from build123d import *

# Parameters (mm, degrees)
F1_DEPTH = 15
F2_R     = 3
F3_R     = 3
F4_R     = 3


with BuildPart() as f1:
    # F0 (on Front) → F1 (new body)
    with BuildSketch(Plane.XZ):
        with BuildLine():
            Line((-16, 27.1340573728), (-16, -16.8659426272))
            Line((-16, -16.8659426272), (-16, -22.8659426272))
            Line((-16, -22.8659426272), (6, -22.8659426272))
            Line((6, -22.8659426272), (6, 27.1340573728))
            Line((6, 27.1340573728), (15, 27.1340573728))
            Line((15, 27.1340573728), (21, 27.1340573728))
            Line((21, 27.1340573728), (21, 49.1340573728))
            Line((21, 49.1340573728), (6, 49.1340573728))
            Line((6, 49.1340573728), (6, 64.1340573728))
            Line((6, 64.1340573728), (0.3713240896, 64.1340573728))
            ThreePointArc((0.3713240896, 64.1340573728), (-5, 58.7627332832), (-10.3713240896, 64.1340573728))
            Line((-10.3713240896, 64.1340573728), (-16, 64.1340573728))
            Line((-16, 64.1340573728), (-16, 49.1340573728))
            Line((-16, 49.1340573728), (-31, 49.1340573728))
            Line((-31, 49.1340573728), (-31, 27.1340573728))
            Line((-31, 27.1340573728), (-25, 27.1340573728))
            Line((-25, 27.1340573728), (-16, 27.1340573728))
        make_face()
        Polygon((-10, 58.1340573728), (0, 58.1340573728), (0, 43.1340573728), (15, 43.1340573728), (15, 33.1340573728), (0, 33.1340573728), (0, -16.8659426272), (-10, -16.8659426272), (-10, 33.1340573728), (-25, 33.1340573728), (-25, 43.1340573728), (-10, 43.1340573728), align=None, mode=Mode.SUBTRACT)
        with BuildLine():
            ThreePointArc((0.3713240896, 64.1340573728), (-5, 69.5053814624), (-10.3713240896, 64.1340573728))
            Line((-10.3713240896, 64.1340573728), (-8.0673756686, 64.1340573728))
            ThreePointArc((-8.0673756686, 64.1340573728), (-5, 67.2014330414), (-1.9326243314, 64.1340573728))
            Line((-1.9326243314, 64.1340573728), (0.3713240896, 64.1340573728))
        make_face()
        with BuildLine():
            Line((-8.0673756686, 64.1340573728), (-10.3713240896, 64.1340573728))
            ThreePointArc((-10.3713240896, 64.1340573728), (-5, 58.7627332832), (0.3713240896, 64.1340573728))
            Line((0.3713240896, 64.1340573728), (-1.9326243314, 64.1340573728))
            ThreePointArc((-1.9326243314, 64.1340573728), (-5, 61.0666817042), (-8.0673756686, 64.1340573728))
        make_face()
    extrude(amount=F1_DEPTH)

    # F2
    f2_edges = [f1.edges().sort_by_distance(p)[0] for p in [
        (-10, -7.5, -16.865943),
        (-10, -7.5, 33.134057),
        (-25, -7.5, 33.134057),
        (0, -7.5, -16.865943),
        (0, -7.5, 33.134057),
        (15, -7.5, 33.134057),
        (15, -7.5, 43.134057),
        (0, -7.5, 43.134057),
        (0, -7.5, 58.134057),
        (-10, -7.5, 58.134057),
        (-10, -7.5, 43.134057),
        (-25, -7.5, 43.134057),
    ]]
    fillet(f2_edges, radius=F2_R)

    # F3
    f3_edges = [f1.edges().sort_by_distance(p)[0] for p in [
        (6, -7.5, 49.134057),
    ]]
    fillet(f3_edges, radius=F3_R)

    # F4
    f4_edges = [f1.edges().sort_by_distance(p)[0] for p in [
        (6, -7.5, 64.134057),
        (0.371324, -7.5, 64.134057),
        (21, -7.5, 27.134057),
        (6, -7.5, 27.134057),
        (6, -7.5, -22.865943),
        (-16, -7.5, -22.865943),
        (-16, -7.5, 27.134057),
        (-31, -7.5, 27.134057),
        (-10.371324, -7.5, 64.134057),
        (-16, -7.5, 64.134057),
        (-16, -7.5, 49.134057),
        (21, -7.5, 49.134057),
        (-31, -7.5, 49.134057),
    ]]
    fillet(f4_edges, radius=F4_R)


solid = f1.part
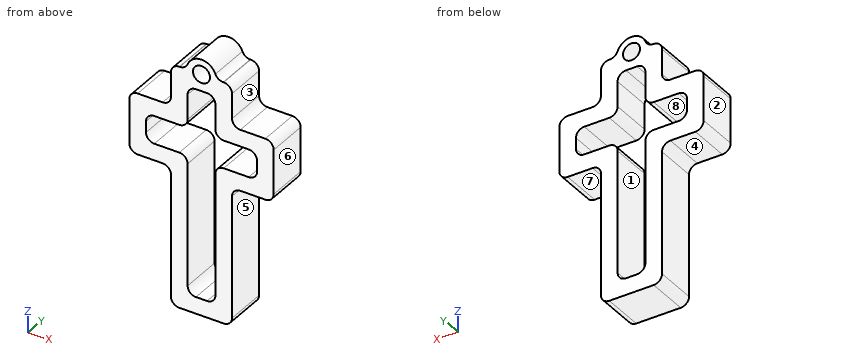
Geometry check sheet. Reference: the model listing, model coordinates, mm. Face numbers are marked on the shaded views. A direction names the side the tool comes from. Give positions to 0.01 mm unless a question says otherwise; leave off trailing zeros. Order: outer loops, then holes, each group sorted by start corner. A loop starts at its lowest first (then second) coordinate and runs counter-clockwise, first axis right, second up. Notation, with made-up numbers: (81, -19) - (98, -19) arc R36 ccw to (98, 16) - close; hole circle Ø1 at (-26.75, -38.75). An arc over 180 degrees is marked (long way). Use one line per item in the form item = value.
1) Sectioned sample at C-C (x = -5). Record the boundary of the cut face in (y, z), and give its area (3 significant figures).
Working result:
outline = (-15, -22.87) - (0, -22.87) - (0, -16.87) - (-15, -16.87) - close; (-15, 58.13) - (0, 58.13) - (0, 61.07) - (-15, 61.07) - close; (-15, 67.2) - (0, 67.2) - (0, 69.51) - (-15, 69.51) - close
area = 169 mm^2
2) Sectioned sample at D-D (y = -8.25). Count the separate pieces of the cut face and the enclosed holes in it, and give its area (3 significant figures).
Working result:
separate_pieces = 1
enclosed_holes = 2
area = 1,540 mm^2
3) Sectioned sample at B-B (x = -21). Record the boundary of the cut face in (y, z), and give its area (3 significant figures).
Working result:
outline = (-15, 27.13) - (0, 27.13) - (0, 33.13) - (-15, 33.13) - close; (-15, 43.13) - (0, 43.13) - (0, 49.13) - (-15, 49.13) - close
area = 180 mm^2
4) Draft check along Z on the marked faces 6, 7 and 8. Enter one of: released by +Z, released by -Z, zero draft, split by the parting line, or undercut.
Working result:
face_6 = zero draft
face_7 = released by -Z
face_8 = undercut
5) Access from +Z, -Z, +X, -X, +Y, -Y to the whole of each face (thin tool, end or side, straight path). Record for the marked faces 1, 2, 3, 4 and 5.
Working result:
face_1 = +Y, -Y
face_2 = +Z, -Z, -X, +Y, -Y
face_3 = +Z, +X, +Y, -Y
face_4 = -Z, -X, +Y, -Y
face_5 = -Z, +X, +Y, -Y
6) Sectioned sample at A-A (z = 21.5). Record the boundary of the cut face in (x, y).
Working result:
outline = (-16, -15) - (-10, -15) - (-10, 0) - (-16, 0) - close; (0, -15) - (6, -15) - (6, 0) - (0, 0) - close
7) Material ranges on probe 1 along Z at (x, y) = (-5, -5.75); probe 2 along X at (y, z) = (-1, 4); probe 3 along X at (y, z) = (-6.5, 36), recorded low to high. Write a range as from..to.
Working result:
probe_1 = -22.87..-16.87, 58.13..61.07, 67.2..69.51
probe_2 = -16..-10, 0..6
probe_3 = -31..-25, 15..21
8) Depth check by flat-ended pin: pin 1 Ø3 at (y, z) = (-9.5, 16) entering from +X; pin 2 Ø7 at (x, y) = (-17.5, -4) entering from +Z; pin 3 Ø3.5 at (x, z) = (-5, 64.13) entering from -Y; pin 4 Ø4 at (x, y) = (14.5, -9.5) entering from +Z. Enter the tip coordinate at first touch or a pass-through.
Working result:
pin_1 = 6
pin_2 = 63.96
pin_3 = through
pin_4 = 49.13
